from build123d import *

# Parameters (mm, degrees)
SKETCH1_W           = 100
SKETCH1_H           = 30
BOSS_EXTRUDE1_DEPTH = 12.7
SKETCH2_W           = 15.2
SKETCH2_H           = 7.62
CUT_EXTRUDE1_DEPTH  = 102.913149299
SKETCH3_W           = 0.635
SKETCH3_H           = 5.08
SKETCH3_W_2         = 10.12
SKETCH3_H_2         = 0.635
CUT_EXTRUDE2_DEPTH  = 102.913149299
BOSS_EXTRUDE2_REACH = 103.913
SKETCH4_W           = 5
SKETCH4_H           = 16.47
FILLET7_R           = 1.5875
FILLET8_R           = 1.5875
BOSS_EXTRUDE3_REACH = 103.405
SKETCH9_W           = 19.05
SKETCH9_H           = 10.12
SKETCH7_R           = 2.54
CUT_EXTRUDE4_DEPTH  = 102.405445613
SKETCH10_R          = 3.175
CUT_EXTRUDE6_DEPTH  = 1.27
FILLET5_R           = 1.5875
BOSS_EXTRUDE4_DEPTH = 12.7
SKETCH12_R          = 4.5
CUT_EXTRUDE7_DEPTH  = 5.08
SKETCH13_R          = 2.75
CUT_EXTRUDE8_DEPTH  = 104.218974152
FILLET6_R           = 5
CUT_EXTRUDE9_START  = -1.27
CUT_EXTRUDE9_DEPTH  = 1.27
SKETCH25_W          = 3.175
SKETCH25_H          = 2.54
BOSS_EXTRUDE5_DEPTH = 2.54
BOSS_EXTRUDE6_REACH = 82.186
SKETCH26_W          = 2.54
SKETCH26_H          = 2.54
SKETCH31_W          = 0.1651
SKETCH31_H          = 2.54
ADJUST_DEPTH        = 72.14
FILLET9_R           = 1.5875
CUT_EXTRUDE10_DEPTH = 104.569962596
FILLET10_R          = 3.81
FILLET11_R          = 2.54


with BuildPart() as part:
    # Sketch1 → Boss-Extrude1 (new body)
    with BuildSketch(Plane(origin=(0, 0, 0), x_dir=(1, 0, 0), z_dir=(0, 1, 0))):
        with Locations((50, 0)):
            Rectangle(SKETCH1_W, SKETCH1_H)
    extrude(amount=BOSS_EXTRUDE1_DEPTH)

    # Sketch2 → Cut-Extrude1 (cut, through all)
    with BuildSketch(Plane(origin=(100, 0, 0), x_dir=(0, 0, -1), z_dir=(1, 0, 0))):
        with Locations((0, 3.81)):
            Rectangle(SKETCH2_W, SKETCH2_H)
    extrude(amount=-CUT_EXTRUDE1_DEPTH, mode=Mode.SUBTRACT)

    # Sketch3 → Cut-Extrude2 (cut, through all)
    with BuildSketch(Plane(origin=(100, 0, 0), x_dir=(0, 0, -1), z_dir=(1, 0, 0))):
        with Locations((-7.9175, 2.54)):
            Rectangle(SKETCH3_W, SKETCH3_H)
        with Locations((0, 7.9375)):
            Rectangle(SKETCH3_W_2, SKETCH3_H_2)
        with Locations((7.9175, 2.54)):
            Rectangle(SKETCH3_W, SKETCH3_H)
    extrude(amount=-CUT_EXTRUDE2_DEPTH, mode=Mode.SUBTRACT)

    # Sketch4 → Boss-Extrude2 (add, up to next)
    with BuildSketch(Plane.XZ, mode=Mode.PRIVATE) as boss_extrude2_sk1:
        with Locations((2.5, 0)):
            Rectangle(SKETCH4_W, SKETCH4_H)
    boss_extrude2_tool1 = extrude(boss_extrude2_sk1.sketch, amount=-BOSS_EXTRUDE2_REACH, mode=Mode.PRIVATE) - part.part
    add(boss_extrude2_tool1.solids().sort_by_distance((2.5, 0, 0))[0])

    # Fillet7
    fillet7_edges = [part.edges().sort_by_distance(p)[0] for p in [
        (5, 6.35, 7.6),
        (5, 6.35, -7.6),
    ]]
    fillet(fillet7_edges, radius=FILLET7_R)

    # Fillet8
    fillet8_edges = [part.edges().sort_by_distance(p)[0] for p in [
        (5, 2.54, 8.235),
        (5, 2.54, -8.235),
    ]]
    fillet(fillet8_edges, radius=FILLET8_R)

    # Sketch9 → Boss-Extrude3 (add, up to next)
    with BuildSketch(Plane.XZ.offset(-7.62), mode=Mode.PRIVATE) as boss_extrude3_sk1:
        with Locations((14.525, 0)):
            Rectangle(SKETCH9_W, SKETCH9_H)
    boss_extrude3_tool1 = extrude(boss_extrude3_sk1.sketch, amount=-BOSS_EXTRUDE3_REACH, mode=Mode.PRIVATE) - part.part
    add(boss_extrude3_tool1.solids().sort_by_distance((14.525, 7.62, 0))[0])

    # Sketch7 → Cut-Extrude4 (cut, through all)
    with BuildSketch(Plane.XZ.offset(-7.62)):
        with Locations(Location((13, 0, 0), (0, 0, 270))):
            Circle(SKETCH7_R)
    extrude(amount=-CUT_EXTRUDE4_DEPTH, mode=Mode.SUBTRACT)

    # Sketch10 → Cut-Extrude6 (cut)
    with BuildSketch(Plane.XZ.offset(-7.62)):
        with Locations(Location((13, 0, 0), (0, 0, 270))):
            Circle(SKETCH10_R)
    extrude(amount=-CUT_EXTRUDE6_DEPTH, mode=Mode.SUBTRACT)

    # Fillet5
    fillet5_edges = [part.edges().sort_by_distance(p)[0] for p in [
        (24.05, 7.9375, 5.06),
        (24.05, 7.9375, -5.06),
    ]]
    fillet(fillet5_edges, radius=FILLET5_R)

    # Sketch11 → Boss-Extrude4 (add)
    with BuildSketch(Plane(origin=(0, 12.7, 0), x_dir=(1, 0, 0), z_dir=(0, 1, 0))):
        with BuildLine():
            Line((68.95, -15), (68.95, -18.415))
            ThreePointArc((68.95, -18.415), (74.95, -24.415), (80.95, -18.415))
            Line((80.95, -18.415), (80.95, -15))
            Line((80.95, -15), (68.95, -15))
        make_face()
        with BuildLine():
            Line((28.51, -18.415), (28.51, -15))
            Line((28.51, -15), (16.51, -15))
            Line((16.51, -15), (16.51, -18.415))
            ThreePointArc((16.51, -18.415), (22.51, -24.415), (28.51, -18.415))
        make_face()
    boss_extrude4 = extrude(amount=-BOSS_EXTRUDE4_DEPTH)

    # Sketch12 → Cut-Extrude7 (cut)
    with BuildSketch(Plane(origin=(0, 12.7, 0), x_dir=(1, 0, 0), z_dir=(0, 1, 0))):
        with Locations(Location((22.51, -18.415, 0), (0, 0, 270))):
            Circle(SKETCH12_R)
        with Locations(Location((74.95, -18.415, 0), (0, 0, 270))):
            Circle(SKETCH12_R)
    cut_extrude7 = extrude(amount=-CUT_EXTRUDE7_DEPTH, mode=Mode.SUBTRACT)

    # Sketch13 → Cut-Extrude8 (cut, through all)
    with BuildSketch(Plane(origin=(0, 7.62, 0), x_dir=(1, 0, 0), z_dir=(0, 1, 0))):
        with Locations(Location((22.51, -18.415, 0), (0, 0, 270))):
            Circle(SKETCH13_R)
        with Locations(Location((74.95, -18.415, 0), (0, 0, 270))):
            Circle(SKETCH13_R)
    cut_extrude8 = extrude(amount=-CUT_EXTRUDE8_DEPTH, mode=Mode.SUBTRACT)

    # Mirror1: Boss-Extrude4, Cut-Extrude7, Cut-Extrude8 across plane
    add(boss_extrude4.mirror(Plane.XY))
    add(cut_extrude7.mirror(Plane.XY), mode=Mode.SUBTRACT)
    add(cut_extrude8.mirror(Plane.XY), mode=Mode.SUBTRACT)

    # Fillet6
    fillet6_edges = [part.edges().sort_by_distance(p)[0] for p in [
        (16.51, 6.35, 15),
        (28.51, 6.35, 15),
        (68.95, 6.35, 15),
        (80.95, 6.35, 15),
        (80.95, 6.35, -15),
        (68.95, 6.35, -15),
        (16.51, 6.35, -15),
        (28.51, 6.35, -15),
    ]]
    fillet(fillet6_edges, radius=FILLET6_R)

    # Sketch24 → Cut-Extrude9 (cut)
    with BuildSketch(Plane.XZ.offset(CUT_EXTRUDE9_START)):
        with BuildLine():
            Line((100, -10.775), (6.5875, -10.775))
            ThreePointArc((6.5875, -10.775), (3.668916761, -9.566083239), (2.46, -6.6475))
            Line((2.46, -6.6475), (2.46, 6.6475))
            ThreePointArc((2.46, 6.6475), (3.668916761, 9.566083239), (6.5875, 10.775))
            Line((6.5875, 10.775), (100, 10.775))
            Line((100, 10.775), (100, 15))
            Line((100, 15), (85.835209001, 15))
            ThreePointArc((85.835209001, 15), (82.564297257, 16.218315671), (80.887386728, 19.279545455))
            ThreePointArc((80.887386728, 19.279545455), (74.95, 24.415), (69.012613272, 19.279545455))
            ThreePointArc((69.012613272, 19.279545455), (67.335702743, 16.218315671), (64.064790999, 15))
            Line((64.064790999, 15), (33.395209001, 15))
            ThreePointArc((33.395209001, 15), (30.124297257, 16.218315671), (28.447386728, 19.279545455))
            ThreePointArc((28.447386728, 19.279545455), (22.51, 24.415), (16.572613272, 19.279545455))
            ThreePointArc((16.572613272, 19.279545455), (14.895702743, 16.218315671), (11.624790999, 15))
            Line((11.624790999, 15), (0, 15))
            Line((0, 15), (0, -15))
            Line((0, -15), (11.624790999, -15))
            ThreePointArc((11.624790999, -15), (14.895702743, -16.218315671), (16.572613272, -19.279545455))
            ThreePointArc((16.572613272, -19.279545455), (22.51, -24.415), (28.447386728, -19.279545455))
            ThreePointArc((28.447386728, -19.279545455), (30.124297257, -16.218315671), (33.395209001, -15))
            Line((33.395209001, -15), (64.064790999, -15))
            ThreePointArc((64.064790999, -15), (67.335702743, -16.218315671), (69.012613272, -19.279545455))
            ThreePointArc((69.012613272, -19.279545455), (74.95, -24.415), (80.887386728, -19.279545455))
            ThreePointArc((80.887386728, -19.279545455), (82.564297257, -16.218315671), (85.835209001, -15))
            Line((85.835209001, -15), (100, -15))
            Line((100, -15), (100, -10.775))
        make_face()
    extrude(amount=CUT_EXTRUDE9_DEPTH, mode=Mode.SUBTRACT)

    # Sketch25 → Boss-Extrude5 (add)
    with BuildSketch(Plane.XZ.offset(-7.62)):
        with Locations((26.2725, 6.33)):
            Rectangle(SKETCH25_W, SKETCH25_H)
        with Locations((26.2725, -6.33)):
            Rectangle(SKETCH25_W, SKETCH25_H)
    extrude(amount=BOSS_EXTRUDE5_DEPTH)

    # Sketch26 → Boss-Extrude6 (add, up to next)
    with BuildSketch(Plane.ZY.offset(-24.685), mode=Mode.PRIVATE) as boss_extrude6_sk1:
        with Locations((6.33, 6.35)):
            Rectangle(SKETCH26_W, SKETCH26_H)
    boss_extrude6_tool1 = extrude(boss_extrude6_sk1.sketch, amount=BOSS_EXTRUDE6_REACH, mode=Mode.PRIVATE) - part.part
    # Sketch26 → Boss-Extrude6 (add, up to next)
    with BuildSketch(Plane.ZY.offset(-24.685), mode=Mode.PRIVATE) as boss_extrude6_sk2:
        with Locations((-6.33, 6.35)):
            Rectangle(SKETCH26_W, SKETCH26_H)
    boss_extrude6_tool2 = extrude(boss_extrude6_sk2.sketch, amount=BOSS_EXTRUDE6_REACH, mode=Mode.PRIVATE) - part.part
    add(boss_extrude6_tool1.solids().sort_by_distance((24.685, 6.35, 6.33))[0])
    add(boss_extrude6_tool2.solids().sort_by_distance((24.685, 6.35, -6.33))[0])

    # Sketch31 → adjust (cut)
    with BuildSketch(Plane(origin=(100, 0, 0), x_dir=(0, 0, -1), z_dir=(1, 0, 0))):
        with Locations((7.68255, 6.35)):
            Rectangle(SKETCH31_W, SKETCH31_H)
        with Locations((-7.68255, 6.35)):
            Rectangle(SKETCH31_W, SKETCH31_H)
    extrude(amount=-ADJUST_DEPTH, mode=Mode.SUBTRACT)

    # Fillet9
    fillet9_edges = [part.edges().sort_by_distance(p)[0] for p in [
        (5, 6.35, 5.06),
        (5, 6.35, -5.06),
        (27.86, 6.35, 7.7651),
        (27.86, 6.35, -7.7651),
    ]]
    fillet(fillet9_edges, radius=FILLET9_R)

    # Sketch33 → Cut-Extrude10 (cut, through all)
    with BuildSketch(Plane.XZ.offset(-1.27)):
        with BuildLine():
            Line((28.447386728, 19.279545455), (28.447386728, 29.295040307))
            Line((28.447386728, 29.295040307), (69.012613272, 29.295040307))
            Line((69.012613272, 29.295040307), (69.012613272, 19.279545455))
            ThreePointArc((69.012613272, 19.279545455), (67.319823601, 15.192789671), (63.233067818, 13.5))
            Line((63.233067818, 13.5), (34.226932182, 13.5))
            ThreePointArc((34.226932182, 13.5), (30.140176399, 15.192789671), (28.447386728, 19.279545455))
        make_face()
        with BuildLine():
            Line((28.447386728, -19.279545455), (28.447386728, -29.295040307))
            Line((28.447386728, -29.295040307), (69.012613272, -29.295040307))
            Line((69.012613272, -29.295040307), (69.012613272, -19.279545455))
            ThreePointArc((69.012613272, -19.279545455), (67.319823601, -15.192789671), (63.233067818, -13.5))
            Line((63.233067818, -13.5), (34.226932182, -13.5))
            ThreePointArc((34.226932182, -13.5), (30.140176399, -15.192789671), (28.447386728, -19.279545455))
        make_face()
    extrude(amount=-CUT_EXTRUDE10_DEPTH, mode=Mode.SUBTRACT)

    # Fillet10
    fillet10_edges = [part.edges().sort_by_distance(p)[0] for p in [
        (0, 6.985, 15),
        (0, 6.985, -15),
    ]]
    fillet(fillet10_edges, radius=FILLET10_R)

    # Fillet11
    fillet11_edges = [part.edges().sort_by_distance(p)[0] for p in [
        (100, 6.985, 15),
        (100, 6.985, -15),
    ]]
    fillet(fillet11_edges, radius=FILLET11_R)


solid = part.part
Read the model definition and answer for the solid it produces. Units are mm, in the model's axes. A direction names the side the tool comes from. Give positions to 0.01 mm unless a question says otherwise; leave off trailing zeros. Write each loop counter-clockwise with the first axis right and the second up, starting at its lowest first coordinate (ties: lowest second). Pieces come first, ordered by that corner, then holes. Notation, with made-up numbers: M 43,24 L 81,24 A15 cw 81,51 Z; hole C -23,-15 d4. An arc over 180 degrees is marked long. One line per item, written item: value. Start each with the question number.
(1) Find section B-B (x = 22.51). Give the number of separate pieces and of enclosed holes in the cut face, plus the area to 3 significant figures.
(2) A tool of negligible diameter and unlimited length cuts with its end or side. For faces 1 (the cylindrical face through (3.701, 0.644, -9.598)), 2 (the flat face through (16, 8.89, 0)), 3 (the flat face through (65, 6, -7.765)), from which of +Z, -Z, +X, -X, +Y, -Y can it reach the whole face along a straight path? Write none if from no direction.
(3) Determine the mould class of faces 4 (the flat face through (65, 6, 7.765)), 5 (the cylindrical face through (22.71, 10.2, -13.92)), 6 (the cylindrical face through (99.276, 7.065, 14.236)) for opening direction X: pulls with the +X half, pulls with the -X half, needs draft (parallel to the pull), parting line crosses it, or undercut.
(4) Flat-ended cylindrical pins translate along their axes: pin 1 Ø4.5 at (x, z) = (75.5, 19.5) entering from +Y; pin 2 Ø2 at (x, z) = (63, 5.5) entering from -Y; pin 3 Ø1 at (x, y) = (46.5, 0.5) entering from -Z (3 decimals). Find the tip coordinate at first contact, or state that the pin passes through.
(5) Find the intervals of material crossed by line 1 (X direction, y = 11.55, z = 0); line 2 (Z direction, x = 95.5, y = 4) (3 decimals); line 3 (X direction, y = 5.25, z = 19.5), in increasing order.
(6) Find section C-C (x = 62). Determine the outline of the cut face in (y, z) (3 decimals).
(7) Find section A-A (z = 0). Determine the outline of the cut face in (x, y) (3 decimals), plus the area to 3 significant figures.
Results below:
1. separate pieces: 3
1. enclosed holes: 0
1. area: 315 mm^2
2. face 1: -Z, -X, -Y
2. face 2: -Y
2. face 3: +X, -Y
3. face 4: needs draft
3. face 5: undercut
3. face 6: pulls with the +X half
4. pin 1: stops at y = 7.62
4. pin 2: stops at y = 7.62
4. pin 3: stops at z = -10.775
5. line 1: x = 0 to 10.46, 15.54 to 100
5. line 2: z = -15 to -8.235, 8.235 to 15
5. line 3: x = 16.61 to 19.98, 25.04 to 28.41, 69.05 to 72.42, 77.48 to 80.85
6. outline: M 0,-10.775 L 1.27,-10.775 L 1.27,-13.5 L 12.7,-13.5 L 12.7,13.5 L 1.27,13.5 L 1.27,10.775 L 0,10.775 L 0,8.235 L 5.08,8.235 L 5.08,7.765 L 7.62,7.765 L 7.62,5.06 L 8.255,5.06 L 8.255,-5.06 L 7.62,-5.06 L 7.62,-7.765 L 5.08,-7.765 L 5.08,-8.235 L 0,-8.235 Z
7. outline: M 0,1.27 L 2.46,1.27 L 2.46,0 L 5,0 L 5,7.62 L 9.825,7.62 L 9.825,8.89 L 10.46,8.89 L 10.46,12.7 L 0,12.7 Z; M 15.54,8.89 L 16.175,8.89 L 16.175,7.62 L 24.05,7.62 L 24.05,8.255 L 100,8.255 L 100,12.7 L 15.54,12.7 Z
7. area: 467 mm^2
